The model under review builds one solid part; all positions refer to its coordinate system, in mm. Face numbers are marked on the shaded views. Round coordinates to 2 decimals unless told otherwise and drop trailing zeros.
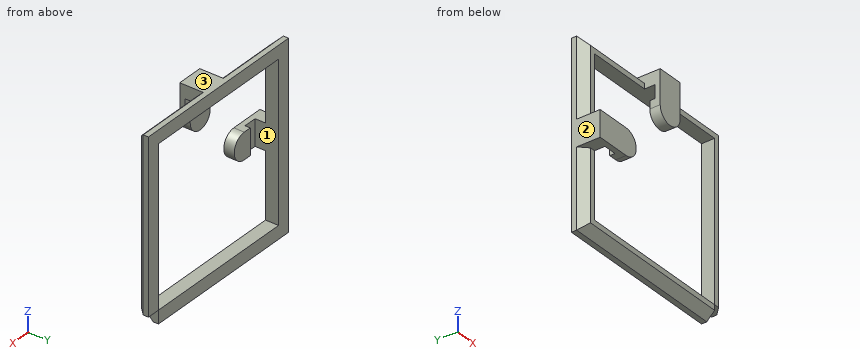
Autodesk Inventor part; units mm, degrees
sketch "Sketch1" plane through (0, 0, 0) normal (0, 1, 0) x (-1, 0, 0)
  line L0 (30, -30) -> (-30, -30)
  line L1 (-30, -30) -> (-30, 30)
  line L2 (-30, 30) -> (30, 30)
  line L3 (30, 30) -> (30, -30)
  line L4 (0, -49.175) -> (0, 49.175)
  line L5 (-49, 0) -> (49, 0)
  line L6 (-35, -35) -> (35, -35)
  line L7 (35, -35) -> (35, 35)
  line L8 (35, 35) -> (-35, 35)
  line L9 (-35, 35) -> (-35, -35)
  line L10 (-30, -30) -> (-30, -35)
  line L11 (-30, -30) -> (-35, -30)
  line L12 (-32, -32) -> (32, -32)
  line L13 (32, -32) -> (32, 32)
  line L14 (32, 32) -> (-32, 32)
  line L15 (-32, 32) -> (-32, -32)
  point P0 (0, 0)
  point P1 (0, -30)
  point P2 (30, 0)
  point P3 (-30, -32)
  point P4 (-32, -30)
  dimension "d0" = 60
  dimension "d1" = 60
  dimension "d2" = 5
  dimension "d3" = 2
extrude "Extrusion1" add sketch "Sketch1" against normal blind 2 contours L12 L13 L5 L7 L6 L4 | L4 L6 L10 L12 | L13 L14 L4 L8 L7 L5 | L11 L9 L5 L15 | L5 L9 L8 L4 L14 L15
extrude "Extrusion2" add sketch "Sketch1" against normal blind 5 contours L3 L5 L13 L12 L4 L0 | L4 L12 L10 L0 | L3 L2 L4 L14 L13 L5 | L11 L15 L5 L1 | L5 L15 L14 L4 L2 L1
chamfer "Chamfer1" distance 3 angle 45 4 edges at (0, -2, 32) (32, -2, 1) (-1, -2, -32) (-32, -2, 0)
sketch "Sketch2" plane through (0, 0, 0) normal (0, 1, 0) x (1, 0, 0)
  line L0 (-30, -30) -> (30, -30)
  line L1 (-35, -35) -> (35, -35)
  line L2 (-5, -30) -> (5, -30)
  line L3 (5, -30) -> (5, -35)
  line L4 (5, -35) -> (-5, -35)
  line L5 (-5, -35) -> (-5, -30)
  line L6 (0, 49.025) -> (0, -49.15)
  point P0 (0, 0)
  point P1 (0, -35)
  dimension "d11" = 10
extrude "Extrusion3" add sketch "Sketch2" against normal blind 11
sketch "Sketch3" plane through (0, -11, 0) normal (0, -1, 0) x (1, 0, 0)
  line L0 (5, 30) -> (30, 30)
  line L1 (5, 30) -> (-5, 30)
  line L2 (-5, 30) -> (-5, 25)
  line L3 (-5, 25) -> (5, 25)
  line L4 (5, 25) -> (5, 30)
  line L5 (-5, 25) -> (5, 25)
  line L6 (5, 25) -> (5, 22)
  line L7 (5, 22) -> (-5, 22)
  line L8 (-5, 22) -> (-5, 25)
  arc A0 (-5, 22) -> (5, 22) centre (0, 22) ccw
  point P0 (0, 0)
  point P1 (5, 25)
  dimension "d14" = 10
  dimension "d15" = 5
  dimension "d16" = 10
  dimension "d17" = 3
extrude "Extrusion4" add sketch "Sketch3" against normal blind 2 contours L4 L3 L2 L1
extrude "Extrusion5" add sketch "Sketch3" against normal blind 4 contours L6 L7 L8 L3 | A0 L7
pattern_circular "Circular Pattern1" count 2 over 90 about axis through (0, -10, 0) along (0, -1, 0) of "Extrusion3", "Extrusion4", "Extrusion5"
properties part number "Marker_Edge"
(1) To check wall thickness, follow probe 1 along Z at (x, y) = (19, -0.75); probe 2 along Z at (x, y) = (-28, -9.25); probe 3 along X at (y, z) = (-3.5, 15.5). State the ranges of each line that lie inside material, in increasing order.
Data:
probe 1: z = -35 to -30, 30 to 35
probe 2: z = -5 to 5
probe 3: x = -33.5 to -30, 30 to 33.5
(2) Draft analysis for pull direction Z (two halves, no side actions). For the marked faces 1, 2 and 3, state which applies: pulls with the +Z half, pulls with the -Z half, needs draft (parallel to the pull), parting line crosses it, or undercut.
Data:
face 1: undercut
face 2: needs draft
face 3: pulls with the +Z half
(3) Insertion check: pin 1 (4 mm diameter, centred on x = 33.5, y = -1.5, fed in from -Z); pin 2 (21.5 mm diameter, centred on x = 4.5, z = -19, fed in from -Y); pin 3 (2.5 mm diameter, centred on y = -5, z = 29, fed in from +X); pin 4 (2.5 mm diameter, centred on y = -4, z = -11.5, fed in from +X). Each pin has a flat end and moves straight along its axis. Give the tip position at first contact, or say it passes through.
Data:
pin 1: stops at z = -30
pin 2: passes through
pin 3: stops at x = 33.25
pin 4: stops at x = 34.25
